Can you work these out from the model? Positions are in its coordinate system, mm. Face numbers are marked on the shaded views. Give positions to 0.01 mm unless a question says otherwise; leave off trailing zeros. Write each loop counter-clockwise with the first axis right and the second up, starting at its lowest first coordinate (ties: lowest second). Pieces come first, ordered by that corner, then holes.
1. Suppose I cut it at A-A (x = 55.5). Please give me the cut outline in (y, z) (1 decimal).
2. Thinking about a two-plate mould opening in Y: for the marked faces 1 and 2, which applies, pulls with the +Y half, pulls with the -Y half, needs draft (parallel to the pull), parting line crosses it, or undercut?
3. If I drill on probe 1 along X at (y, z) = (1, -3.5); probe 2 along X at (y, z) = (-2.75, -3.5); probe 3 along Z at (x, y) = (41.5, 3.75), over which ranges is the centre line in solid material (lowest first)?
4. I'm going to push flat-ended pins straight in: pin 1 (5 mm diameter, centred on y = 0.5, z = -0.5, fed in from -X); pin 2 (1.5 mm diameter, centred on x = 38.5, z = -1, fed in from -Y). Where does each tip first touch, or does it pass through?
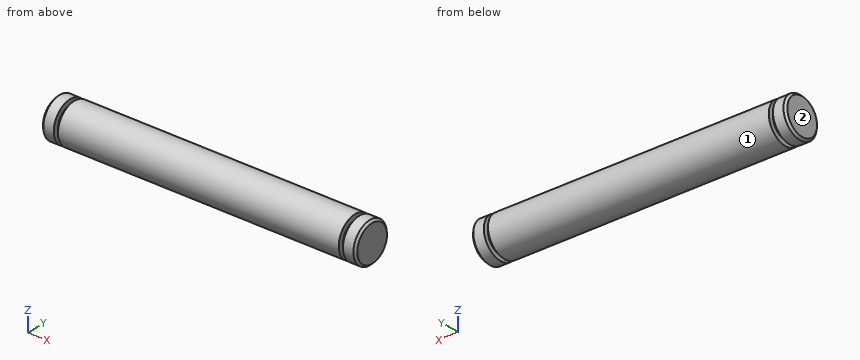
Autodesk Inventor part; units mm, degrees
ref_plane "YZ Plane" through (0, 0, 0) normal (1, 0, 0) x (0, 1, 0)
ref_plane "XZ Plane" through (0, 0, 0) normal (0, 1, 0) x (-1, 0, 0)
ref_plane "XY Plane" through (0, 0, 0) normal (0, 0, 1) x (1, 0, 0)
sketch "Esboço2" plane through (0, 0, 0) normal (1, 0, 0) x (0, 1, 0)
  circle A0 centre (0, 0) radius 4.7625
  dimension "d0" = 9.525
extrude "Extrusão1" add sketch "Esboço2" along normal blind 3
sketch "Esboço3" plane through (3, 0, 0) normal (1, 0, 0) x (0, 0, -1)
  circle A0 centre (0, 0) radius 4.7625
  circle A1 centre (0, 0) radius 3.5719
  dimension "d3" = 7.1437
extrude "Extrusão2" add sketch "Esboço3" along normal blind 1 contours A1
sketch "Esboço4" plane through (4, 0, 0) normal (1, 0, 0) x (0, 0, -1)
  circle A0 centre (0, 0) radius 3.5719
  circle A1 centre (0, 0) radius 4.7625
  dimension "d6" = 9.525
extrude "Extrusão3" add sketch "Esboço4" along normal blind 67 contours A0 | A1
sketch "Esboço5" plane through (71, 0, 0) normal (1, 0, 0) x (0, 0, -1)
  circle A0 centre (0, 0) radius 4.7625
  circle A1 centre (0, 0) radius 3.5719
  dimension "d9" = 7.1437
extrude "Extrusão4" add sketch "Esboço5" along normal blind 1 contours A1
sketch "Esboço6" plane through (72, 0, 0) normal (1, 0, 0) x (0, 0, -1)
  circle A0 centre (0, 0) radius 3.5719
  circle A1 centre (0, 0) radius 4.7625
  dimension "d12" = 9.525
extrude "Extrusão5" add sketch "Esboço6" along normal blind 3 contours A0 | A1
chamfer "Chanfro1" distance 0.5 angle 45 2 edges at (0, -4.7625, 0) (75, 0, 4.7625)
properties part number "pino_a3" material "Aço carbono"
Checks:
1. outline: circle Ø9.5 at (0, 0)
2. face 1: parting line crosses it
2. face 2: needs draft
3. probe 1: x = 0 to 3, 4 to 71, 72 to 75
3. probe 2: x = 0.19 to 3, 4 to 71, 72 to 74.81
3. probe 3: z = -2.94 to 2.94
4. pin 1: stops at x = 0
4. pin 2: stops at y = -4.76
